from build123d import *

# Parameters (mm, degrees)
F0_W          = 38.25
F0_H          = 3
F1_DEPTH      = 1.5
F2_DEPTH      = 1.5
F5_DEPTH      = 0.75
F6_R          = 1.5
F7_W          = 1.5
F7_H          = 71.928761142
F8_DEPTH      = 17.5
F10_SIZE      = 3
F13_R         = 1.75
F14_DEPTH     = 25
F15_DEPTH     = 1
F16_T4_DEPTH  = 48.5367319519
F16_T10_DEPTH = 48.5367319519
F16_T15_DEPTH = 80.0367319519
F16_T22_DEPTH = 40.0367319519
F16_T27_DEPTH = 40.0367319519


# Not quite as in the source:
# - a fillet or chamfer that OpenCascade refuses, or shapes differently, is made with other operations: its cross-section is extruded or revolved along the edge and cut away or added


with BuildPart() as f1:
    # F0 (on Top) → F1 (new body)
    with BuildSketch(Plane.XY):
        with BuildLine():
            Line((-14, -42.5426968038), (-23.75, -42.5426968038))
            Line((-23.75, -42.5426968038), (-23.75, -42.9965845553))
            Line((-23.75, -42.9965845553), (-21.0181723213, -43.3122070099))
            ThreePointArc((-21.0181723213, -43.3122070099), (-18.8056300503, -44.4619063855), (-17.919875499, -46.7926982744))
            Line((-17.919875499, -46.7926982744), (-17.9227195281, -49.5426968038))
            Line((-17.9227195281, -49.5426968038), (15.75, -49.5426968038))
            Line((15.75, -49.5426968038), (15.75, -42.5426968038))
            Line((15.75, -42.5426968038), (-14, -42.5426968038))
        make_face()
        with BuildLine():
            Line((18, 49.2073031962), (-17.5, 49.2073031962))
            Line((-17.5, 49.2073031962), (-17.5, 46.4573031962))
            ThreePointArc((-17.5, 46.4573031962), (-18.5251262658, 43.982429462), (-21, 42.9573031962))
            Line((-21, 42.9573031962), (-23.75, 42.9573031962))
            Line((-23.75, 42.9573031962), (-23.75, -42.5426968038))
            Line((-23.75, -42.5426968038), (-14, -42.5426968038))
            Line((-14, -42.5426968038), (-14, 26.2073031962))
            Line((-14, 26.2073031962), (-14, 29.2073031962))
            Line((-14, 29.2073031962), (24.25, 29.2073031962))
            Line((24.25, 29.2073031962), (24.25, 42.9570424259))
            Line((24.25, 42.9570424259), (21.4996681305, 42.9573032119))
            ThreePointArc((21.4996681305, 42.9573032119), (19.0250089351, 43.9825467984), (18, 46.4573031962))
            Line((18, 46.4573031962), (18, 49.2073031962))
        make_face()
        with Locations((5.125, 27.7073031962)):
            Rectangle(F0_W, F0_H)
    extrude(amount=F1_DEPTH)

    # F0 (on Top) → F2 (join)
    with BuildSketch(Plane.XY):
        with BuildLine():
            Line((-14, -42.5426968038), (-23.75, -42.5426968038))
            Line((-23.75, -42.5426968038), (-23.75, -42.9965845553))
            Line((-23.75, -42.9965845553), (-21.0181723213, -43.3122070099))
            ThreePointArc((-21.0181723213, -43.3122070099), (-18.8056300503, -44.4619063855), (-17.919875499, -46.7926982744))
            Line((-17.919875499, -46.7926982744), (-17.9227195281, -49.5426968038))
            Line((-17.9227195281, -49.5426968038), (15.75, -49.5426968038))
            Line((15.75, -49.5426968038), (15.75, -42.5426968038))
            Line((15.75, -42.5426968038), (-14, -42.5426968038))
        make_face()
        with Locations((5.125, 27.7073031962)):
            Rectangle(F0_W, F0_H)
    extrude(amount=-F2_DEPTH)

    # F3: union 

    # F4 (on face) → F5 (cut)
    with BuildSketch(Plane.XY):
        Polygon((-19.8072306812, 41.2358827889), (-27.7905139636, 41.2358827889), (-27.9461211857, -15.0937307626), (-19.8072306812, -15.0937307626), align=None)
    extrude(amount=F5_DEPTH, mode=Mode.SUBTRACT)

    # F6
    f6_edges = [f1.edges().sort_by_distance(p)[0] for p in [
        (-17.5, 49.207303, 0.75),
        (-23.75, 42.957303, 0.75),
        (18, 49.207303, 0.75),
        (24.25, 42.957042, 0.75),
        (-23.75, -42.996585, 0),
        (-17.92272, -49.542697, 0),
    ]]
    fillet(f6_edges, radius=F6_R)

    # F7 (on Top) → F8 (join)
    with BuildSketch(Plane.XY):
        with Locations((-14.7299332246, -6.7935563562)):
            Rectangle(F7_W, F7_H)
    extrude(amount=-F8_DEPTH)

    # F9: union 

    # F10
    f10_edges = [f1.edges().sort_by_distance(p)[0] for p in [
        (-14.729933, -42.757937, -17.5),
        (-14.729933, 29.170824, -17.5),
    ]]
    chamfer(f10_edges, length=F10_SIZE)


with BuildPart() as f11_1:
    # F11: copy of F1
    add(f1.part)


with BuildPart() as f1_1:
    add(f1.part)

    # F13 (on face) → F14 (cut)
    with BuildSketch(Plane.XY.offset(1.5)):
        with Locations((5.438e-07, 35.8340851963)):
            Circle(F13_R)
    extrude(amount=-F14_DEPTH, mode=Mode.SUBTRACT)

    # F15 (cut): a face of the model
    f15_faces = [f1_1.faces().sort_by_distance(p)[0] for p in [
        (0.8800150014, -42.5426968038, 0.0002530279),
    ]]
    extrude(f15_faces, amount=-F15_DEPTH, mode=Mode.SUBTRACT)

    # F16: chamfer of 2 on 3 edges, made by hand


with BuildPart() as f16_tool2:
    # F16_s3 → F16_t4 (new body)
    with BuildSketch(Plane.YZ.offset(-19.1433659759)):
        Polygon((28.2073031962, 1.5), (26.2073031962, -0.5), (26.2073031962, 1.5), align=None)
    extrude(amount=F16_T4_DEPTH)

    split(bisect_by=Plane.XY, keep=Keep.TOP)

    split(bisect_by=Plane(origin=(-7.25, 0, -7.25), x_dir=(0, 1, 0), z_dir=(0.7071067812, 0, 0.7071067812)), keep=Keep.TOP)


with BuildPart() as f1_2:
    add(f1_1.part)

    # F16_t1: cut F16_tool2
    add(f16_tool2.part, mode=Mode.SUBTRACT)


with BuildPart() as f16_tool8:
    # F16_s9 → F16_t10 (new body)
    with BuildSketch(Plane.YZ.offset(-19.1433659759)):
        Polygon((28.2073031962, 1.5), (26.2073031962, -0.5), (26.2073031962, 1.5), align=None)
    extrude(amount=F16_T10_DEPTH)

    split(bisect_by=Plane.YZ.offset(-13.9799332246), keep=Keep.TOP)


with BuildPart() as f1_3:
    add(f1_2.part)

    # F16_t7: cut F16_tool8
    add(f16_tool8.part, mode=Mode.SUBTRACT)


with BuildPart() as f16_tool13:
    # F16_s14 → F16_t15 (new body)
    with BuildSketch(Plane.XZ.offset(48.6860627797)):
        Polygon((-14, -0.5), (-16, 1.5), (-14, 1.5), align=None)
    extrude(amount=-F16_T15_DEPTH)

    split(bisect_by=Plane.XY, keep=Keep.TOP)

    split(bisect_by=Plane(origin=(0, 13.3536515981, -13.3536515981), x_dir=(1, 0, 0), z_dir=(0, -0.7071067812, 0.7071067812)), keep=Keep.TOP)

    split(bisect_by=Plane(origin=(0, -22.0213484019, -22.0213484019), x_dir=(1, 0, 0), z_dir=(0, 0.7071067812, 0.7071067812)), keep=Keep.TOP)


with BuildPart() as f1_4:
    add(f1_3.part)

    # F16_t12: cut F16_tool13
    add(f16_tool13.part, mode=Mode.SUBTRACT)


with BuildPart() as f16_tool20:
    # F16_s21 → F16_t22 (new body)
    with BuildSketch(Plane.YZ.offset(20.8933659759)):
        Polygon((-43.5426968038, -0.5), (-45.5426968038, 1.5), (-43.5426968038, 1.5), align=None)
    extrude(amount=-F16_T22_DEPTH)

    split(bisect_by=Plane.YZ.offset(-13.9799332246), keep=Keep.TOP)


with BuildPart() as f1_5:
    add(f1_4.part)

    # F16_t19: cut F16_tool20
    add(f16_tool20.part, mode=Mode.SUBTRACT)


with BuildPart() as f16_tool25:
    # F16_s26 → F16_t27 (new body)
    with BuildSketch(Plane.YZ.offset(20.8933659759)):
        Polygon((-43.5426968038, -0.5), (-45.5426968038, 1.5), (-43.5426968038, 1.5), align=None)
    extrude(amount=-F16_T27_DEPTH)

    split(bisect_by=Plane.XY, keep=Keep.TOP)

    split(bisect_by=Plane(origin=(-7.25, 0, -7.25), x_dir=(0, 1, 0), z_dir=(0.7071067812, 0, 0.7071067812)), keep=Keep.TOP)


with BuildPart() as f1_6:
    add(f1_5.part)

    # F16_t24: cut F16_tool25
    add(f16_tool25.part, mode=Mode.SUBTRACT)


solid = f1_6.part
Can you work these out from the model? Positions are in its coordinate system, mm. A direction names the side the tool comes from. Give positions to 0.01 mm unless a question says otherwise; leave off trailing zeros. Loops run counter-clockwise (first coordinate to the right, second up) from the corner with the lowest first, then second, coordinate; pieces in that order, holes last. Notation, with made-up numbers: (73, 75.5) -> (113, 75.5) arc R26 cw to (113, 101.5) -> close; hole circle Ø2 at (52.25, -17.5). An arc over 180 degrees is marked (long way). Write item = value, one per line.
1) Will these pins go through, and if not, where does the flat tip stop? pin 1 (2 mm diameter, centred on x = -22.5, y = 4, fed in from -Z); pin 2 (10 mm diameter, centred on y = 5.5, z = -2.5, fed in from +X); pin 3 (3.5 mm diameter, centred on x = 3.5, y = -45.5, fed in from -Z).
Check result:
pin_1 = 0.75
pin_2 = -13.98
pin_3 = -1.5
2) For faces 1 (the flat face through (3.84, 27.22, 0.51)), 2 (the flat face through (15.75, -47, 0)), 3 (the flat face through (-22, 13, 0.75)), which set-ups out of +Z, -Z, +X, -X, +Y, -Y let a thin tool reach every point of the face, with its end or its side?
Check result:
face_1 = +Z, +X
face_2 = +Z, -Z, +X, -Y
face_3 = -Z, -X
3) Suppose I cut it at D-D on z = -3. Write out the boundary of the cut face in (x, y), then the cut area to 3 significant figures.
Check result:
outline = (-15.48, -42.76) -> (-13.98, -42.76) -> (-13.98, 29.17) -> (-15.48, 29.17) -> close
area = 108 mm2
4) Thinking about a two-plate mould opening in Y: for faces 4 (the flat face through (-16, 21, 0)), 5 (the flat face through (0.1, -44.53, 0.49)), 6 (the cylindrical face through (19.05, 43.96, 0.74)), which applies, released by +Y, released by -Y, zero draft, split by the parting line, or undercut?
Check result:
face_4 = zero draft
face_5 = undercut
face_6 = released by +Y
5) I need wall thicknesses on L1, parallel to Y at x = 9, z = -1.25; L2, parallel to Y at x = 0, z = 0.5; L3, parallel to Y at x = 0, z = 1. Which ranges of each line are inside material? Lowest first, please. Write a range as from..to.
Check result:
L1 = -49.54..-43.54, 26.21..29.21
L2 = -49.54..-44.54, 27.21..34.08, 37.58..49.21
L3 = -49.54..-45.04, 27.71..34.08, 37.58..49.21
6) Suppose I cut it at A-A on x = -13. Write out the boundary of the cut face in (y, z), then the cut area to 3 significant figures.
Check result:
outline = (-49.54, -1.5) -> (-43.54, -1.5) -> (-43.54, -0.5) -> (-45.54, 1.5) -> (-49.54, 1.5) -> close; (26.21, -1.5) -> (29.21, -1.5) -> (29.21, 0) -> (49.21, 0) -> (49.21, 1.5) -> (28.21, 1.5) -> (26.21, -0.5) -> close
area = 53.0 mm2
7) Suppose I cut it at C-C on x = 0.5. Write out the boundary of the cut face in (y, z).
Check result:
outline = (-49.54, -1.5) -> (-43.54, -1.5) -> (-43.54, -0.5) -> (-45.54, 1.5) -> (-49.54, 1.5) -> close; (26.21, -1.5) -> (29.21, -1.5) -> (29.21, 0) -> (34.16, 0) -> (34.16, 1.5) -> (28.21, 1.5) -> (26.21, -0.5) -> close; (37.51, 0) -> (49.21, 0) -> (49.21, 1.5) -> (37.51, 1.5) -> close
8) Suppose I cut it at B-B on y = 5.5. Write out the boundary of the cut face in (x, z), then the cut area to 3 significant figures.
Check result:
outline = (-23.75, 0.75) -> (-19.81, 0.75) -> (-19.81, 0) -> (-15.48, 0) -> (-15.48, -17.5) -> (-13.98, -17.5) -> (-13.98, 0) -> (-14.5, 0) -> (-16, 1.5) -> (-23.75, 1.5) -> close
area = 36.0 mm2
